Design review of the part built by this model. Coordinates are the model's own, in mm. A direction names the side the tool comes from. Coordinates: 2 decimals unless noted, no trailing zeros. Write each loop counter-clockwise with the first axis right and the second up, starting at its lowest first coordinate (ties: lowest second). Pieces come first, ordered by that corner, then holes.
Autodesk Inventor part; units mm, degrees
ref_plane "COMBINATION_MODULE_XY" through (0, 0, 0.3) normal (0, 0, 1) x (1, 0, 0)
ref_plane "COMBINATION_MODULE_YZ" through (0, 0, 0.3) normal (1, 0, 0) x (0, 1, 0)
ref_plane "COMBINATION_MODULE_ZX" through (0, 0, 0.3) normal (0, 1, 0) x (0, 0, 1)
sketch "Sketch_1" plane through (0, 0, 0) normal (0, 0, 1) x (1, 0, 0)
  arc A0 (3.1835, -4.485) -> (-3.1835, -4.485) centre (0, 0) ccw
  line L0 (-3.1835, -4.485) -> (-2.15, -1.2757)
  arc A1 (-2.5, 0) -> (-2.15, -1.2757) centre (0, 0) ccw
  line L1 (-2.5, 0) -> (-4.3, 0)
  arc A2 (-1.4, 4.0657) -> (-4.3, 0) centre (0, 0) ccw
  line L2 (-1.4, 4.0657) -> (-1.0001, 2.2912)
  arc A3 (1.0001, 2.2912) -> (-1.0001, 2.2912) centre (0, 0) ccw
  line L3 (1.0001, 2.2912) -> (1.4, 4.0657)
  arc A4 (4.3, 0) -> (1.4, 4.0657) centre (0, 0) ccw
  line L4 (4.3, 0) -> (2.5, 0)
  arc A5 (2.15, -1.2757) -> (2.5, 0) centre (0, 0) ccw
  line L5 (2.15, -1.2757) -> (3.1835, -4.485)
extrude "Extrusion1" add sketch "Sketch_1" along normal mid plane 0.6
ref_plane "COMBINATION_MODULE_XY" through (0, 0, 0.3) normal (0, 0, 1) x (1, 0, 0)
ref_plane "COMBINATION_MODULE_YZ" through (0, 0, 0.3) normal (1, 0, 0) x (0, 1, 0)
ref_plane "COMBINATION_MODULE_ZX" through (0, 0, 0.3) normal (0, 1, 0) x (0, 0, 1)
ref_plane "ring_to_screw_XY" through (0, 0, 0) normal (0, 0, 1) x (1, 0, 0)
ref_plane "ring_to_screw_YZ" through (0, 0, 0) normal (1, 0, 0) x (0, 1, 0)
ref_plane "ring_to_screw_ZX" through (0, 0, 0) normal (0, 1, 0) x (0, 0, 1)
properties part number "NETW5"
(1) Mouldability with a two-part tool opening along X and no side actions: class faces 4 (the flat face through (0, 3, 0.3)), 5 (the cylindrical face through (-0.194, 5.497, -0.004)), 6 (the cylindrical face through (-3.5, 2.5, 0)) as +X half, -X half, draft (parallel to the pull), parting line (faces both ways), or undercut.
(2) Consider section A-A (y = 3.25). Give the boundary of the cut face in (x, z).
(3) Consider section B-B (y = 1.25). Give the boundary of the cut face in (x, z).
(4) Wall thickness on line 1 (X direction, y = 2, z = 0.1); line 2 (Y direction, x = -3.25, z = -0.1); line 3 (X direction, y = 3.5, z = 0.2): over which ranges is each line inside the solid? List them lowest first.
(5) For faces 1 (the flat face through (0, 3, -0.3)), 2 (the flat face through (-2.674, -2.903, -0.004)), 3 (the cylindrical face through (3.5, 2.5, 0)), list the 3-axis set-ups (+Z, -Z, +X, -X, +Y, -Y) from which the entire face can be reached by the end or side of a thin tool; tool diameter is ignored.
(6) Consider section D-D (x = 3). Give the boundary of the cut face in (y, z).
Results:
1. face 4: draft
1. face 5: parting line
1. face 6: undercut
2. outline: (-4.44, -0.3) - (-2.82, -0.3) - (-2.82, 0.3) - (-4.44, 0.3) - close; (-1.22, -0.3) - (1.22, -0.3) - (1.22, 0.3) - (-1.22, 0.3) - close; (2.82, -0.3) - (4.44, -0.3) - (4.44, 0.3) - (2.82, 0.3) - close
3. outline: (-5.36, -0.3) - (-4.11, -0.3) - (-4.11, 0.3) - (-5.36, 0.3) - close; (4.11, -0.3) - (5.36, -0.3) - (5.36, 0.3) - (4.11, 0.3) - close
4. line 1: x = -5.12 to -3.81, 3.81 to 5.12
4. line 2: y = -4.44 to 0, 2.82 to 4.44
4. line 3: x = -4.24 to -2.5, -1.27 to 1.27, 2.5 to 4.24
5. face 1: -Z, +X, -X, +Y, -Y
5. face 2: +Z, -Z, -Y
5. face 3: +Z, -Z
6. outline: (-3.92, -0.3) - (0, -0.3) - (0, 0.3) - (-3.92, 0.3) - close; (3.08, -0.3) - (4.61, -0.3) - (4.61, 0.3) - (3.08, 0.3) - close
